```python
from build123d import *

# Parameters (mm, degrees)
BOSS_EXTRUDE1_DEPTH                           = 2.54
CSK_FOR_4_FLAT_HEAD_MACHINE_SCREW1_AT_2_COUNT = 2
CSK_FOR_4_FLAT_HEAD_MACHINE_SCREW1_AT_2_PITCH = 50.8
CSK_FOR_4_FLAT_HEAD_MACHINE_SCREW1_AT_3_COUNT = 2
CSK_FOR_4_FLAT_HEAD_MACHINE_SCREW1_AT_3_PITCH = 86.36933773
CSK_FOR_4_FLAT_HEAD_MACHINE_SCREW1_AT_4_COUNT = 2
CSK_FOR_4_FLAT_HEAD_MACHINE_SCREW1_AT_4_PITCH = 69.85
SKETCH5_W                                     = 36.59505
SKETCH5_H                                     = 27.305
BOSS_EXTRUDE2_DEPTH                           = 15.24
CUT_EXTRUDE2_REACH                            = 58.398
SKETCH8_R                                     = 2.0193
FILLET1_R                                     = 2.54
CUT_EXTRUDE4_DEPTH                            = 3.429
FILLET2_R                                     = 3.175
SKETCH10_W                                    = 25.4
SKETCH10_H                                    = 8.255
CUT_EXTRUDE5_DEPTH                            = 57.398148028
FILLET3_R                                     = 1.27


with BuildPart() as part:
    # Sketch1 → Boss-Extrude1 (new body)
    with BuildSketch(Plane(origin=(0, 0, 0), x_dir=(1, 0, 0), z_dir=(0, 1, 0))):
        with BuildLine():
            Line((-36.5125, 30.1625), (36.5125, 30.1625))
            ThreePointArc((36.5125, 30.1625), (38.75756403, 29.23256403), (39.6875, 26.9875))
            Line((39.6875, 26.9875), (39.6875, -26.9875))
            ThreePointArc((39.6875, -26.9875), (38.75756403, -29.23256403), (36.5125, -30.1625))
            Line((36.5125, -30.1625), (-36.5125, -30.1625))
            ThreePointArc((-36.5125, -30.1625), (-38.75756403, -29.23256403), (-39.6875, -26.9875))
            Line((-39.6875, -26.9875), (-39.6875, 26.9875))
            ThreePointArc((-39.6875, 26.9875), (-38.75756403, 29.23256403), (-36.5125, 30.1625))
        make_face()
    extrude(amount=BOSS_EXTRUDE1_DEPTH)

    # Sketch3 → CSK for #4 Flat Head Machine Screw1 (revolve, cut)
    with BuildSketch(Plane(origin=(-34.925, 2.54, -25.4), x_dir=(0, 0, 1), z_dir=(1, 0, 0))):
        Polygon((0, 0), (0, 2.54), (1.63195, 2.54), (1.63195, 1.848124365), (3.2385, 0), align=None)
    csk_for_4_flat_head_machine_screw1 = revolve(axis=Axis((-34.925, 8.89, -25.4), (0, -1, 0)), mode=Mode.SUBTRACT)

    # CSK for #4 Flat Head Machine Screw1 at 2: CSK for #4 Flat Head Machine Screw1 ×2
    with Locations(*[(0, 0, i * CSK_FOR_4_FLAT_HEAD_MACHINE_SCREW1_AT_2_PITCH) for i in range(1, CSK_FOR_4_FLAT_HEAD_MACHINE_SCREW1_AT_2_COUNT)]):
        add(csk_for_4_flat_head_machine_screw1, mode=Mode.SUBTRACT)

    # CSK for #4 Flat Head Machine Screw1 at 3: CSK for #4 Flat Head Machine Screw1 ×2
    with Locations(*[Vector(0.8087360843031886, 0, 0.5881716976750463) * (i * CSK_FOR_4_FLAT_HEAD_MACHINE_SCREW1_AT_3_PITCH) for i in range(1, CSK_FOR_4_FLAT_HEAD_MACHINE_SCREW1_AT_3_COUNT)]):
        add(csk_for_4_flat_head_machine_screw1, mode=Mode.SUBTRACT)

    # CSK for #4 Flat Head Machine Screw1 at 4: CSK for #4 Flat Head Machine Screw1 ×2
    with Locations(*[(i * CSK_FOR_4_FLAT_HEAD_MACHINE_SCREW1_AT_4_PITCH, 0, 0) for i in range(1, CSK_FOR_4_FLAT_HEAD_MACHINE_SCREW1_AT_4_COUNT)]):
        add(csk_for_4_flat_head_machine_screw1, mode=Mode.SUBTRACT)

    # Sketch5 → Boss-Extrude2 (add)
    with BuildSketch(Plane(origin=(0, 2.54, 0), x_dir=(1, 0, 0), z_dir=(0, 1, 0))):
        with Locations((0, -9.8425)):
            Rectangle(SKETCH5_W, SKETCH5_H)
    extrude(amount=BOSS_EXTRUDE2_DEPTH)

    # Sketch4 → Cut-Revolve1 (revolve, cut)
    with BuildSketch(Plane(origin=(0, 0, 0), x_dir=(0, 0, -1), z_dir=(1, 0, 0))):
        Polygon((-32.244261254, 22.052492284), (-6.188048119, 48.10870542), (12.054444166, 29.866213135), (-14.00176897, 3.81), align=None)
    revolve(axis=Axis((0, 29.866213135, -12.054444166), (0, 0.7071067811865511, 0.707106781186544)), mode=Mode.SUBTRACT)

    # Cut-Extrude2: up to this plane
    cut_extrude2_end = Plane(origin=(-18.297525, 17.78, -3.81), z_dir=(0, 0, 1))
    # Sketch8 → Cut-Extrude2 (cut, up to the surface)
    with BuildSketch(Plane(origin=(0, 8.905884485, 8.905884485), x_dir=(1, 0, 0), z_dir=(0, 0.7071067811865511, 0.707106781186544)), mode=Mode.PRIVATE) as cut_extrude2_sk1:
        with Locations(Location((-12.7, 9.195689, 0), (0, 0, 270))):
            Circle(SKETCH8_R)
    cut_extrude2_tool1 = split(extrude(cut_extrude2_sk1.sketch, amount=-CUT_EXTRUDE2_REACH, mode=Mode.PRIVATE), bisect_by=cut_extrude2_end, keep=Keep.BOTH, mode=Mode.PRIVATE)
    add(cut_extrude2_tool1.solids().sort_by_distance((-12.7, 15.408219, 2.40355))[0], mode=Mode.SUBTRACT)
    # Sketch8 → Cut-Extrude2 (cut, up to the surface)
    with BuildSketch(Plane(origin=(0, 8.905884485, 8.905884485), x_dir=(1, 0, 0), z_dir=(0, 0.7071067811865511, 0.707106781186544)), mode=Mode.PRIVATE) as cut_extrude2_sk2:
        with Locations(Location((12.7, 9.195689, 0), (0, 0, 270))):
            Circle(SKETCH8_R)
    cut_extrude2_tool2 = split(extrude(cut_extrude2_sk2.sketch, amount=-CUT_EXTRUDE2_REACH, mode=Mode.PRIVATE), bisect_by=cut_extrude2_end, keep=Keep.BOTH, mode=Mode.PRIVATE)
    add(cut_extrude2_tool2.solids().sort_by_distance((12.7, 15.408219, 2.40355))[0], mode=Mode.SUBTRACT)

    # Fillet1
    # the kernel refuses this fillet: 2.54 mm, written as the material it takes off along each edge
    with BuildSketch(Plane(origin=(18.297525, 2.54, -3.81), x_dir=(-1, 0, 0), z_dir=(0, 1, 0)), Plane(origin=(18.297525, 2.54, 23.495), x_dir=(0, 0, -1), z_dir=(0, 1, 0)), Plane(origin=(-18.297525, 2.54, 23.495), x_dir=(1, 0, 0), z_dir=(0, 1, 0))) as fillet1_piece_1:
        with BuildLine():
            CenterArc((FILLET1_R, FILLET1_R), FILLET1_R, 180, 90)
            Line((0, FILLET1_R), (0, 0))
            Line((0, 0), (FILLET1_R, 0))
        make_face()
    extrude(amount=21.59, mode=Mode.SUBTRACT)
    with BuildSketch(Plane(origin=(-18.297525, 2.54, -3.81), x_dir=(1, 0, 0), z_dir=(0, 1, 0))) as fillet1_piece_2:
        with BuildLine():
            CenterArc((FILLET1_R, -FILLET1_R), FILLET1_R, 90, 90)
            Line((0, -FILLET1_R), (0, 0))
            Line((0, 0), (FILLET1_R, 0))
        make_face()
    extrude(amount=21.59, mode=Mode.SUBTRACT)
    # the kernel refuses this fillet: 2.54 mm, written as the material it adds along each edge
    with BuildSketch(Plane(origin=(-15.757525, 2.54, -3.81), x_dir=(0, 0, -1), z_dir=(1, 0, 0)), Plane(origin=(15.757525, 2.54, 23.495), x_dir=(0, 0, 1), z_dir=(-1, 0, 0))) as fillet1_2_piece_1:
        with BuildLine():
            CenterArc((FILLET1_R, FILLET1_R), FILLET1_R, 180, 90)
            Line((0, FILLET1_R), (0, 0))
            Line((0, 0), (FILLET1_R, 0))
        make_face()
    extrude(amount=31.51505)
    with BuildSketch(Plane(origin=(18.297525, 2.54, -1.27), x_dir=(1, 0, 0), z_dir=(0, 0, 1)), Plane(origin=(-18.297525, 2.54, 20.955), x_dir=(-1, 0, 0), z_dir=(0, 0, -1))) as fillet1_2_piece_2:
        with BuildLine():
            CenterArc((FILLET1_R, FILLET1_R), FILLET1_R, 180, 90)
            Line((0, FILLET1_R), (0, 0))
            Line((0, 0), (FILLET1_R, 0))
        make_face()
    extrude(amount=22.225)
    with BuildSketch(Plane(origin=(-15.757525, 2.54, 20.955), x_dir=(0, 0, 1), z_dir=(1, 0, 0))) as fillet1_2_piece_3:
        with BuildLine():
            CenterArc((2.54 + FILLET1_R, -FILLET1_R), FILLET1_R, 90, 90)
            Line((2.54, -FILLET1_R), (2.54, 0))
            Line((2.54, 0), (2.54 + FILLET1_R, 0))
        make_face()
    revolve(axis=Axis((-15.757525, 2.54, 20.955), (0, -1, 0)), revolution_arc=90)
    with BuildSketch(Plane(origin=(-15.757525, 2.54, -1.27), x_dir=(0, 0, -1), z_dir=(1, 0, 0))) as fillet1_2_piece_4:
        with BuildLine():
            CenterArc((2.54 + FILLET1_R, FILLET1_R), FILLET1_R, 180, 90)
            Line((2.54, FILLET1_R), (2.54, 0))
            Line((2.54, 0), (2.54 + FILLET1_R, 0))
        make_face()
    revolve(axis=Axis((-15.757525, 2.54, -1.27), (0, 1, 0)), revolution_arc=90)
    with BuildSketch(Plane(origin=(15.757525, 2.54, 20.955), x_dir=(1, 0, 0), z_dir=(0, 0, -1))) as fillet1_2_piece_5:
        with BuildLine():
            CenterArc((2.54 + FILLET1_R, -FILLET1_R), FILLET1_R, 90, 90)
            Line((2.54, -FILLET1_R), (2.54, 0))
            Line((2.54, 0), (2.54 + FILLET1_R, 0))
        make_face()
    revolve(axis=Axis((15.757525, 2.54, 20.955), (0, -1, 0)), revolution_arc=90)
    with BuildSketch(Plane(origin=(15.757525, 2.54, -1.27), x_dir=(0, 0, -1), z_dir=(-1, 0, 0))) as fillet1_2_piece_6:
        with BuildLine():
            CenterArc((2.54 + FILLET1_R, -FILLET1_R), FILLET1_R, 90, 90)
            Line((2.54, -FILLET1_R), (2.54, 0))
            Line((2.54, 0), (2.54 + FILLET1_R, 0))
        make_face()
    revolve(axis=Axis((15.757525, 2.54, -1.27), (0, -1, 0)), revolution_arc=90)

    # Sketch9 → Cut-Extrude4 (cut)
    with BuildSketch(Plane(origin=(0, 2.54, 0), x_dir=(1, 0, 0), z_dir=(0, 1, 0))):
        with BuildLine():
            Line((-30.677270284, 30.1625), (30.677270284, 30.1625))
            Line((30.677270284, 30.1625), (14.939561121, 18.716893336))
            ThreePointArc((14.939561121, 18.716893336), (0, 13.858789877), (-14.939561121, 18.716893336))
            Line((-14.939561121, 18.716893336), (-30.677270284, 30.1625))
        make_face()
        with BuildLine():
            Line((-39.6875, 20.6375), (-39.6875, -20.6375))
            ThreePointArc((-39.6875, -20.6375), (-25.711391971, 0), (-39.6875, 20.6375))
        make_face()
        with BuildLine():
            Line((39.6875, 20.6375), (39.6875, -20.6375))
            ThreePointArc((39.6875, -20.6375), (25.711391971, 0), (39.6875, 20.6375))
        make_face()
        with BuildLine():
            Line((-30.677270284, -30.1625), (30.677270284, -30.1625))
            ThreePointArc((30.677270284, -30.1625), (0, -26.401718952), (-30.677270284, -30.1625))
        make_face()
    extrude(amount=-CUT_EXTRUDE4_DEPTH, mode=Mode.SUBTRACT)

    # Fillet2
    fillet2_edges = [part.edges().sort_by_distance(p)[0] for p in [
        (-39.6875, 1.27, -20.6375),
        (-39.6875, 1.27, 20.6375),
        (-30.677270284, 1.27, 30.1625),
        (30.677270284, 1.27, 30.1625),
        (39.6875, 1.27, 20.6375),
        (39.6875, 1.27, -20.6375),
        (30.677270284, 1.27, -30.1625),
        (-30.677270284, 1.27, -30.1625),
    ]]
    fillet(fillet2_edges, radius=FILLET2_R)

    # Sketch10 → Cut-Extrude5 (cut, through all)
    with BuildSketch(Plane(origin=(0, 8.905884485, 8.905884485), x_dir=(1, 0, 0), z_dir=(0, 0.7071067811865529, 0.7071067811865422))):
        with Locations((0, -0.1378966)):
            Rectangle(SKETCH10_W, SKETCH10_H)
    extrude(amount=-CUT_EXTRUDE5_DEPTH, mode=Mode.SUBTRACT)

    # Fillet3
    fillet3_edges = [part.edges().sort_by_distance(p)[0] for p in [
        (12.7, 5.863480052, 0.221328815),
        (12.7, 2.944896812, 8.977078533),
        (-12.7, 2.944896812, 8.977078533),
        (-12.7, 5.863480052, 0.221328815),
    ]]
    fillet(fillet3_edges, radius=FILLET3_R)


solid = part.part
```
Build history of the part. All positions in model axes, mm. A direction names the side the tool comes from. Give positions to 0.01 mm unless a question says otherwise; leave off trailing zeros. Loops run counter-clockwise (first coordinate to the right, second up) from the corner with the lowest first, then second, coordinate; pieces in that order, holes last. Notation, with made-up numbers: (-11.75, 31.5) -> (0.25, 31.5) arc R4 cw to (0.25, 37.5) -> close; hole circle Ø10 at (59.25, -21). An arc over 180 degrees is marked (long way). One line per question, with ' | ' between items.
Q1. Drill centre lines: line 1 along X through (y, z) = (0.3, 25.4); line 2 along X through (y, z) = (0.55, -25.4); line 3 along Z through (x, y) = (-16, 10.25). Where is each one in solid material? Low to high. Write a range as [from, to].
Filled sheet:
line 1: x = [-39.69, -36.56], [-33.29, 33.29], [36.56, 39.69] | line 2: x = [-39.69, -36.56], [-33.29, -24.13], [24.13, 33.29], [36.56, 39.69] | line 3: z = [-3.8, 7.56], [15.27, 23.48]
Q2. Drop flat-ended pins along their axis: pin 1 (4 mm diameter, centred on y = 12.5, z = 7, fed in from -X); pin 2 (10 mm diameter, centred on y = 10, z = 12, fed in from +X); pin 3 (5.5 mm diameter, centred on y = 4, z = 2.5, fed in from -X); pin 4 (1.5 mm diameter, centred on x = -9, z = -6.5, fed in from -Y). Give the stop position or say it passes through.
Filled sheet:
pin 1: stops at x = -18.3 | pin 2: stops at x = 18.3 | pin 3: stops at x = -26.24 | pin 4: stops at y = 0
Q3. Cut at A-A, the plane z = -25.4. Write the cut outline in (x, y).
Filled sheet:
outline: (-39.69, 0) -> (-36.56, 0) -> (-36.56, 0.69) -> (-38.16, 2.54) -> (-39.69, 2.54) -> close; (-33.29, 0) -> (-24.13, 0) -> (-24.13, 2.54) -> (-31.69, 2.54) -> (-33.29, 0.69) -> close; (24.13, 0) -> (33.29, 0) -> (33.29, 0.69) -> (31.69, 2.54) -> (24.13, 2.54) -> close; (36.56, 0) -> (39.69, 0) -> (39.69, 2.54) -> (38.16, 2.54) -> (36.56, 0.69) -> close
Q4. Tool access for faces 1 (the cylindrical face through (-39.228, 1.252, -21.042)), 2 (the cylindrical face through (-30.71, 1.25, -30)), 3 (the flat face through (12.7, 5, 5)): list every direction of +Z, -Z, +X, -X, +Y, -Y with a clear straight run to the whole face (end or side of a thin tool).
Filled sheet:
face 1: -X, +Y, -Y | face 2: -Z, +Y, -Y | face 3: none
Q5. Pull direction X, two halves, no side cores. Call faces 4 (the cylindrical face through (38.78, 1.25, 29.21)), 5 (the flat face through (0, 11, -3.81)), 6 (the cylindrical face through (0.22, 1.29, -13.86)): pulls with the +X half, pulls with the -X half, needs draft (parallel to the pull), parting line crosses it, or undercut.
Filled sheet:
face 4: pulls with the +X half | face 5: needs draft | face 6: undercut
Q6. Cut at B-B, the plane x = -7. Write the cut outline in (y, z) (3 decimals).
Filled sheet:
outline: (0, -14.842) -> (2.54, -14.842) -> (2.54, -6.35) arc R2.54 cw to (5.08, -3.81) -> (17.78, -3.81) -> (17.78, 0.032) -> (11.727, 6.085) -> (0, -5.642) -> close; (0, 6.032) -> (5.89, 11.922) -> (4.284, 13.527) -> (14.252, 23.495) -> (5.08, 23.495) arc R2.54 cw to (2.54, 26.035) -> (2.54, 26.595) -> (0, 26.595) -> close
